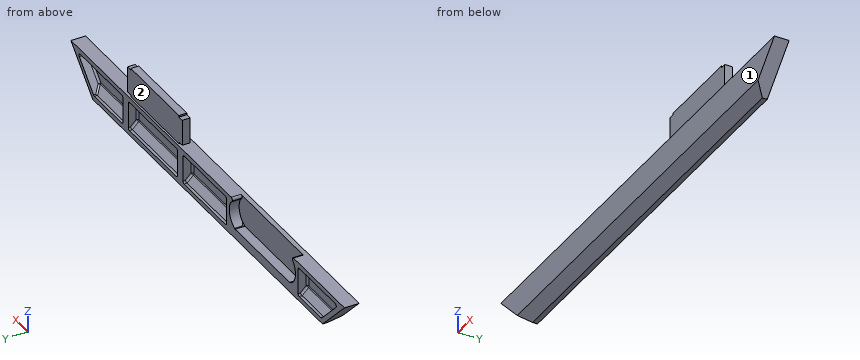
from build123d import *

# Parameters (mm, degrees)
BOSS_EXTRUDE1_DEPTH     = 3.75
SKETCH3_W               = 50
SKETCH3_H               = 15
BOSS_EXTRUDE3_DEPTH     = 4
CUT_EXTRUDE1_DEPTH      = 128.641098397
CUT_EXTRUDE1_DEPTH_BACK = 4
CHAMFER1_SIZE           = 5
SKETCH7_W               = 3
SKETCH7_H               = 0.853193318
CUT_EXTRUDE2_DEPTH      = 128.641098397
SHELL1_START            = -17.283882181
SHELL1_DEPTH            = 121.248348275
SHELL1_START_2          = -103.964466094
SHELL1_2_DEPTH          = 21.248348275
SHELL1_START_3          = -118.964466094
SHELL1_3_DEPTH          = 43.546786157
SHELL1_START_4          = -24.582320063
SHELL1_4_DEPTH          = 143.546786157
SHELL1_START_5          = -1.25
SHELL1_5_DEPTH          = 5
BOSS_EXTRUDE4_REACH     = 129.696
RIB1_REACH              = 129.696
SKETCH5_WALLS_W         = 5
SKETCH5_WALLS_H         = 272.391855782
FILLET1_R               = 1
FILLET3_R               = 1


with BuildPart() as part:
    # Sketch1 → Boss-Extrude1 (new, symmetric)
    with BuildSketch(Plane(origin=(0, 0, 0), x_dir=(1, 0, 0), z_dir=(0, 1, 0))):
        Polygon((-125, -10), (125, -10), (105, 10), (-105, 10), align=None)
    extrude(amount=BOSS_EXTRUDE1_DEPTH, both=True)

    # Sketch3 → Boss-Extrude3 (add)
    with BuildSketch(Plane(origin=(0, 2.75, 0), x_dir=(-1, 0, 0), z_dir=(0, 1, 0))):
        with Locations((-50, 17.5)):
            Rectangle(SKETCH3_W, SKETCH3_H)
    extrude(amount=-BOSS_EXTRUDE3_DEPTH)

    # Sketch4 → Cut-Extrude1 (cut, two sides: drawn at the far end of the back side and taken through both)
    with BuildSketch(Plane(origin=(0, 2.75, 0), x_dir=(-1, 0, 0), z_dir=(0, 1, 0)).offset(-CUT_EXTRUDE1_DEPTH_BACK)):
        with BuildLine():
            Line((75, 10), (25, 10))
            ThreePointArc((25, 10), (19.783882181, 2.5), (25, -5))
            Line((25, -5), (75, -5))
            ThreePointArc((75, -5), (80.216117819, 2.5), (75, 10))
        make_face()
    extrude(amount=CUT_EXTRUDE1_DEPTH + CUT_EXTRUDE1_DEPTH_BACK, mode=Mode.SUBTRACT)

    # Chamfer1
    chamfer1_edges = [part.edges().sort_by_distance(p)[0] for p in [
        (0, -3.75, -10),
    ]]
    chamfer(chamfer1_edges, length=CHAMFER1_SIZE)

    # Sketch7 → Cut-Extrude2 (cut, through all)
    with BuildSketch(Plane(origin=(0, 2.75, 0), x_dir=(-1, 0, 0), z_dir=(0, 1, 0))):
        with Locations((-73.5, 24.573403341)):
            Rectangle(SKETCH7_W, SKETCH7_H)
        with Locations((-73.5, 10.426596659)):
            Rectangle(SKETCH7_W, SKETCH7_H)
        with Locations((-26.5, 10.426596659)):
            Rectangle(SKETCH7_W, SKETCH7_H)
        with Locations((-26.5, 24.573403341)):
            Rectangle(SKETCH7_W, SKETCH7_H)
    extrude(amount=-CUT_EXTRUDE2_DEPTH, mode=Mode.SUBTRACT)

    # Shell1: read off the stored shape, not the designer's step
    # Shell1 outline → Shell1 (cut)
    with BuildSketch(Plane.YZ.offset(SHELL1_START)):
        Polygon((-1.25, 7.5), (-1.25, -3.964466094), (2.285533906, -7.5), (3.75, -7.5), (3.75, 7.5), align=None)
    extrude(amount=SHELL1_DEPTH, mode=Mode.SUBTRACT)

    # Shell1 2 outline → Shell1 2 (cut)
    with BuildSketch(Plane.YZ.offset(SHELL1_START_2)):
        Polygon((-1.25, 7.5), (-1.25, -3.964466094), (2.285533906, -7.5), (3.75, -7.5), (3.75, 7.5), align=None)
    extrude(amount=SHELL1_2_DEPTH, mode=Mode.SUBTRACT)

    # Shell1 3 outline → Shell1 3 (cut)
    with BuildSketch(Plane.YZ.offset(SHELL1_START_3)):
        Polygon((-1.25, 7.5), (-1.25, -3.964466094), (2.285533906, -7.5), (3.75, -7.5), (3.75, 7.5), align=None)
    extrude(amount=SHELL1_3_DEPTH, mode=Mode.SUBTRACT)

    # Shell1 4 outline → Shell1 4 (cut)
    with BuildSketch(Plane.YZ.offset(SHELL1_START_4)):
        Polygon((-1.25, 7.5), (-1.25, -3.964466094), (2.285533906, -7.5), (3.75, -7.5), (3.75, 7.5), align=None)
    extrude(amount=SHELL1_4_DEPTH, mode=Mode.SUBTRACT)

    # Shell1 5 outline → Shell1 5 (add)
    with BuildSketch(Plane(origin=(0, 0, 0), x_dir=(1, 0, 0), z_dir=(0, 1, 0)).offset(SHELL1_START_5)):
        Polygon((-107.5, 7.5), (-118.964466094, -3.964466094), (-118.964466094, -7.5), (-103.964466094, 7.5), align=None)
        with BuildLine():
            ThreePointArc((-75.417679937, 7.5), (-81.958045751, 1.417249055), (-81.449210475, -7.5))
            Line((-81.449210475, -7.5), (-78.461115817, -7.5))
            ThreePointArc((-78.461115817, -7.5), (-79.983065249, -0.58309426), (-75.417679937, 4.831439149))
            Line((-75.417679937, 4.831439149), (-75.417679937, 7.5))
        make_face()
        Polygon((118.964466094, -3.964466094), (107.5, 7.5), (103.964466094, 7.5), (118.964466094, -7.5), align=None)
        with BuildLine():
            ThreePointArc((-18.550789525, -7.5), (-18.041954249, 1.417249055), (-24.582320063, 7.5))
            Line((-24.582320063, 7.5), (-24.582320063, 4.831439149))
            ThreePointArc((-24.582320063, 4.831439149), (-20.016934751, -0.58309426), (-21.538884183, -7.5))
            Line((-21.538884183, -7.5), (-18.550789525, -7.5))
        make_face()
    extrude(amount=SHELL1_5_DEPTH)

    # Sketch6 → Boss-Extrude4 (add, up to next)
    with BuildSketch(Plane.XZ.offset(-3.75), mode=Mode.PRIVATE) as boss_extrude4_sk1:
        with BuildLine():
            Line((-17.283882181, -7.5), (-17.283882181, 2.500000029))
            ThreePointArc((-17.283882181, 2.500000029), (-19.302537873, -3.69005644), (-24.582320063, -7.5))
            Line((-24.582320063, -7.5), (-17.283882181, -7.5))
        make_face()
    boss_extrude4_tool1 = extrude(boss_extrude4_sk1.sketch, amount=BOSS_EXTRUDE4_REACH, mode=Mode.PRIVATE) - part.part
    # Sketch6 → Boss-Extrude4 (add, up to next)
    with BuildSketch(Plane.XZ.offset(-3.75), mode=Mode.PRIVATE) as boss_extrude4_sk2:
        with BuildLine():
            Line((-17.283882181, 2.500000029), (-17.283882181, 7.5))
            Line((-17.283882181, 7.5), (-18.550789525, 7.5))
            ThreePointArc((-18.550789525, 7.5), (-17.605535736, 5.079004387), (-17.283882181, 2.500000029))
        make_face()
    boss_extrude4_tool2 = extrude(boss_extrude4_sk2.sketch, amount=BOSS_EXTRUDE4_REACH, mode=Mode.PRIVATE) - part.part
    # Sketch6 → Boss-Extrude4 (add, up to next)
    with BuildSketch(Plane.XZ.offset(-3.75), mode=Mode.PRIVATE) as boss_extrude4_sk3:
        with BuildLine():
            Line((-82.716117819, 7.5), (-82.716117819, 2.499999956))
            ThreePointArc((-82.716117819, 2.499999956), (-82.394464273, 5.079004351), (-81.449210475, 7.5))
            Line((-81.449210475, 7.5), (-82.716117819, 7.5))
        make_face()
    boss_extrude4_tool3 = extrude(boss_extrude4_sk3.sketch, amount=BOSS_EXTRUDE4_REACH, mode=Mode.PRIVATE) - part.part
    # Sketch6 → Boss-Extrude4 (add, up to next)
    with BuildSketch(Plane.XZ.offset(-3.75), mode=Mode.PRIVATE) as boss_extrude4_sk4:
        with BuildLine():
            Line((-82.716117819, -7.5), (-75.417679937, -7.5))
            ThreePointArc((-75.417679937, -7.5), (-80.697462105, -3.69005647), (-82.716117819, 2.499999956))
            Line((-82.716117819, 2.499999956), (-82.716117819, -7.5))
        make_face()
    boss_extrude4_tool4 = extrude(boss_extrude4_sk4.sketch, amount=BOSS_EXTRUDE4_REACH, mode=Mode.PRIVATE) - part.part
    add(boss_extrude4_tool1.solids().sort_by_distance((-19.229077, 3.75, -5.202593))[0])
    add(boss_extrude4_tool2.solids().sort_by_distance((-17.659672, 3.75, 6.265582))[0])
    add(boss_extrude4_tool3.solids().sort_by_distance((-82.340328, 3.75, 6.265582))[0])
    add(boss_extrude4_tool4.solids().sort_by_distance((-80.770923, 3.75, -5.202593))[0])

    # Sketch5 walls → Rib1 (add, up to next)
    with BuildSketch(Plane.XZ.offset(-3.75), mode=Mode.PRIVATE) as rib1_sk1:
        with Locations((75, 0)):
            Rectangle(SKETCH5_WALLS_W, SKETCH5_WALLS_H)
    rib1_tool1 = extrude(rib1_sk1.sketch, amount=RIB1_REACH, mode=Mode.PRIVATE) - part.part
    # Sketch5 walls → Rib1 (add, up to next)
    with BuildSketch(Plane.XZ.offset(-3.75), mode=Mode.PRIVATE) as rib1_sk2:
        with Locations((25, 0)):
            Rectangle(SKETCH5_WALLS_W, SKETCH5_WALLS_H)
    rib1_tool2 = extrude(rib1_sk2.sketch, amount=RIB1_REACH, mode=Mode.PRIVATE) - part.part
    add(rib1_tool1.solids().sort_by_distance((75, 3.75, 0))[0])
    add(rib1_tool2.solids().sort_by_distance((25, 3.75, 0))[0])

    # Fillet1
    fillet1_edges = [part.edges().sort_by_distance(p)[0] for p in [
        (113.232233047, -1.25, 1.767766953),
        (105.732233047, 0.517766953, -5.732233047),
        (118.964466094, 1.25, 7.5),
        (103.964466094, 3.017766953, -7.5),
        (-103.964466094, 3.017766953, -7.5),
        (-105.732233047, 0.517766953, -5.732233047),
        (-113.232233047, -1.25, 1.767766953),
        (-100.840291956, -1.25, 7.5),
        (-118.964466094, 1.25, 7.5),
        (-95.108058909, -1.25, -3.964466094),
        (2.608058909, -1.25, -3.964466094),
        (-17.283882181, -1.25, 1.767766953),
        (-17.283882181, 0.517766953, -5.732233047),
        (-17.283882181, 3.017766953, -7.5),
        (2.608058909, -1.25, 7.5),
        (-17.283882181, 1.25, 7.5),
        (-82.716117819, -1.25, 1.767766953),
        (-82.716117819, 1.25, 7.5),
        (-82.716117819, 0.517766953, -5.732233047),
        (-82.716117819, 3.017766953, -7.5),
        (92.5, -1.25, -3.964466094),
        (77.5, 0.517766953, -5.732233047),
        (72.5, 0.517766953, -5.732233047),
        (98.232233047, -1.25, 7.5),
        (72.5, 1.25, 7.5),
        (77.5, -1.25, 1.767766953),
        (72.5, -1.25, 1.767766953),
        (72.5, 3.017766953, -7.5),
        (77.5, 1.25, 7.5),
        (77.5, 3.017766953, -7.5),
        (50, -1.25, -3.964466094),
        (27.5, 0.517766953, -5.732233047),
        (22.5, 0.517766953, -5.732233047),
        (50, -1.25, 7.5),
        (27.5, -1.25, 1.767766953),
        (22.5, 1.25, 7.5),
        (22.5, -1.25, 1.767766953),
        (22.5, 3.017766953, -7.5),
        (27.5, 1.25, 7.5),
        (27.5, 3.017766953, -7.5),
    ]]
    fillet(fillet1_edges, radius=FILLET1_R)

    # Fillet3
    fillet3_edges = [part.edges().sort_by_distance(p)[0] for p in [
        (-25, 1.25, 10),
        (-25, 1.25, -5),
        (-75, 1.25, -5),
        (-75, 1.25, 10),
    ]]
    fillet(fillet3_edges, radius=FILLET3_R)


solid = part.part
The model under review builds one solid part; all positions refer to its coordinate system, in mm. Face numbers are marked on the shaded views. A direction names the side the tool comes from. Give positions to 0.01 mm unless a question says otherwise; leave off trailing zeros. Order: outer loops, then holes, each group sorted by start corner. A loop starts at its lowest first (then second) coordinate and runs counter-clockwise, first axis right, second up. Notation, with made-up numbers: M 34.5,51.25 L 75.5,51.25 A21 cw 75.5,86.25 Z; hole C -7.5,-5 d2. An arc over 180 degrees is marked long. Answer in a Markdown table with one row per item. Add a question column.
1. Add section D-D on z = 13. State the section outline as (x, y) points, plus the area to 3 significant figures.
2. Add section C-C on x = -44.5. State the section outline as (y, z) points.
3. To check wall thickness, follow line 1 along Z through (x, y) = (97, 3.25); line 2 along X through (y, z) = (2.25, 6); line 3 along Z through (x, y) = (69.5, 2.5). State the ranges of each line that lie inside material, in increasing order.
4. Add section A-A on x = 59. State the section outline as (y, z) points, plus the area to 3 significant figures.
5. Add section B-B on y = -2.5. State the section outline as (x, z) points.
6. For pin 1 Ø0.9 at (y, z) = (1.5, 10.5) entering from +X; pin 2 Ø1.5 at (x, y) = (73, 0.5) entering from +Z; pin 3 Ø7.5 at (x, z) = (-37, 5) entering from +Y, all flat-tipped, find the tip position at first contact; note any pin that passes through.
7. Machinability: for the marked faces 1 and 2, which of the approach directions +Z, -Z, +X, -X, +Y, -Y give a long, thin tool a straight path to every point of the face, cutting with its end or side? Answer none if there is none.
The answers:
| question | item | result |
|---|---|---|
| 1 | outline | M 25,-1.25 L 75,-1.25 L 75,2.75 L 25,2.75 Z |
| 1 | area | 200 mm2 |
| 2 | outline | M -3.75,-5 L 1.25,-10 L 3.75,-10 L 3.75,-5 L -1.25,-5 L -1.25,10 L -3.75,10 Z |
| 3 | line 1 | -10 to -7.5, 7.5 to 10 |
| 3 | line 2 | -121 to -117.42, -82.72 to -79.41, -20.59 to -17.28, 22.5 to 27.5, 72.5 to 77.5, 117.42 to 121 |
| 3 | line 3 | -10 to -7.5, 7.5 to 25 |
| 4 | outline | M -3.75,-5 L 1.25,-10 L 3.75,-10 L 3.75,-7.5 L 2.29,-7.5 L -0.96,-4.26 A1 cw -1.25,-3.55 L -1.25,6.5 A1 cw -0.25,7.5 L 3.75,7.5 L 3.75,10 L 2.75,10 L 2.75,25 L -1.25,25 L -1.25,10 L -3.75,10 Z |
| 4 | area | 129 mm2 |
| 5 | outline | M -125,10 L -108.75,-6.25 L 108.75,-6.25 L 125,10 Z |
| 6 | pin 1 | x = 75 |
| 6 | pin 2 | z = 24.15 |
| 6 | pin 3 | y = -1.25 |
| 7 | face 1 | +Z, -Z, +X, -X, -Y |
| 7 | face 2 | +Z, +X, -X, +Y |
